Read the model definition and answer for the solid it produces. Units are mm, in the model's axes. A direction names the side the tool comes from. Coordinates: 2 decimals unless noted, no trailing zeros. Order: outer loops, then holes, each group sorted by start corner. A loop starts at its lowest first (then second) coordinate and runs counter-clockwise, first axis right, second up. Notation, with made-up numbers: M 86.5,72.25 L 131.5,72.25 A24 ccw 131.5,107.25 Z; hole C 29,68.5 d4. An arc over 180 degrees is marked long. Write each question's results on one line, items separated by ' | '.
```python
from build123d import *

# Parameters (mm, degrees)
BOSS_EXTRUDE1_DEPTH           = 10
M4_CLEARANCE_HOLE1_AT_2_COUNT = 2
M4_CLEARANCE_HOLE1_AT_2_PITCH = 112
SKETCH6_R                     = 3
CUT_EXTRUDE1_DEPTH            = 8
CUT_EXTRUDE1_DEPTH_BACK       = 6
FILLET1_R                     = 1


with BuildPart() as part:
    # Sketch1 → Boss-Extrude1 (new body)
    with BuildSketch(Plane(origin=(0, 0, 0), x_dir=(0, 0, -1), z_dir=(1, 0, 0))):
        with BuildLine():
            ThreePointArc((25, 57.609374237), (12.766583292, 61.488652214), (0, 62.8))
            ThreePointArc((0, 62.8), (-12.766583292, 61.488652214), (-25, 57.609374237))
            Line((-25, 57.609374237), (-25, 51.929182547))
            ThreePointArc((-25, 51.929182547), (-25.220795702, 51.145833095), (-25.818181818, 50.593097233))
            ThreePointArc((-25.818181818, 50.593097233), (-43.035646203, 37.069841595), (-53.859344034, 18.039153533))
            ThreePointArc((-53.859344034, 18.039153533), (-54.405495004, 17.298046479), (-55.281685866, 17.01553963))
            Line((-55.281685866, 17.01553963), (-59.5, 17.01553963))
            ThreePointArc((-59.5, 17.01553963), (-60.560660172, 16.576199802), (-61, 15.51553963))
            Line((-61, 15.51553963), (-61, 2.01553963))
            Line((-61, 2.01553963), (-50.76, 2.01553963))
            ThreePointArc((-50.76, 2.01553963), (0, 50.8), (50.76, 2.01553963))
            Line((50.76, 2.01553963), (61, 2.01553963))
            Line((61, 2.01553963), (61, 15.51553963))
            ThreePointArc((61, 15.51553963), (60.560660172, 16.576199802), (59.5, 17.01553963))
            Line((59.5, 17.01553963), (55.281685866, 17.01553963))
            ThreePointArc((55.281685866, 17.01553963), (54.405495004, 17.298046479), (53.859344034, 18.039153533))
            ThreePointArc((53.859344034, 18.039153533), (43.035646203, 37.069841595), (25.818181818, 50.593097233))
            ThreePointArc((25.818181818, 50.593097233), (25.220795702, 51.145833095), (25, 51.929182547))
            Line((25, 51.929182547), (25, 57.609374237))
        make_face()
    extrude(amount=BOSS_EXTRUDE1_DEPTH)

    # Sketch4 → M4 Clearance Hole1 (revolve, cut)
    with BuildSketch(Plane(origin=(5, 17.01553963, -56), x_dir=(0, 0, 1), z_dir=(1, 0, 0))):
        Polygon((0, 0), (0, 16.351936393), (2.25, 15), (2.25, 0), align=None)
    m4_clearance_hole1 = revolve(axis=Axis((5, 23.36553963, -56), (0, -1, 0)), mode=Mode.SUBTRACT)

    # M4 Clearance Hole1 at 2: M4 Clearance Hole1 ×2
    with Locations(*[(0, 0, i * M4_CLEARANCE_HOLE1_AT_2_PITCH) for i in range(1, M4_CLEARANCE_HOLE1_AT_2_COUNT)]):
        add(m4_clearance_hole1, mode=Mode.SUBTRACT)

    # Sketch6 → Cut-Extrude1 (cut, two sides)
    with BuildSketch(Plane(origin=(0, 17.01553963, 0), x_dir=(1, 0, 0), z_dir=(0, 1, 0))) as cut_extrude1_sk:
        with Locations((5, 56)):
            Circle(SKETCH6_R)
        with Locations((5, -56)):
            Circle(SKETCH6_R)
    extrude(amount=CUT_EXTRUDE1_DEPTH, mode=Mode.SUBTRACT)
    extrude(cut_extrude1_sk.sketch, amount=-CUT_EXTRUDE1_DEPTH_BACK, mode=Mode.SUBTRACT)

    # Fillet1
    fillet1_edges = [part.edges().sort_by_distance(p)[0] for p in [
        (5, 57.609374237, -25),
        (5, 57.609374237, 25),
    ]]
    fillet(fillet1_edges, radius=FILLET1_R)


solid = part.part
```
(1) The part is cut by section C-C, the plane y = 23.5. Write down the section's boundary in (x, z), then the cut area to 3 significant figures.
Conclusion:
outline: M 0,-51.71 L 10,-51.71 L 10,-45.04 L 0,-45.04 Z; M 0,45.04 L 10,45.04 L 10,51.71 L 0,51.71 Z | area: 133 mm²
(2) Given pin 1 (3 mm diameter, centred on x = 4, z = 57, fed in from +Y); pin 2 (8 mm diameter, centred on y = 32.5, z = 44, fed in from -X); pin 3 (1 mm diameter, centred on x = 2, z = -20.5, fed in from +Y); pin 4 (5.5 mm diameter, centred on x = 2.5, y = 53.5, fed in from -Z), each flat-ended and moving along its own axis, determine where each tip first touches the part or whether it passes through.
Conclusion:
pin 1: y = 11.02 | pin 2: x = 0 | pin 3: y = 59.53 | pin 4: z = -25.57
(3) The mould has two halves that part along X. Classify faces 4 (the cylindrical face through (4.901, 6.579, -58.248)), 5 (the flat face through (0, 51, 9)), 6 (the flat face through (2.7, 2.016, 54.8)), 7 (the flat face through (10, 51, 9)): pulls with the +X half, pulls with the -X half, needs draft (parallel to the pull), parting line crosses it, or undercut.
Conclusion:
face 4: undercut | face 5: pulls with the -X half | face 6: needs draft | face 7: pulls with the +X half
(4) The part is cut by section B-B, the plane y = 40. Write down the section's boundary in (x, z).
Conclusion:
outline: M 0,-40.33 L 10,-40.33 L 10,-31.32 L 0,-31.32 Z; M 0,31.32 L 10,31.32 L 10,40.33 L 0,40.33 Z
(5) For faces 1 (the cylindrical face through (4.901, 6.579, 53.752)), 2 (the flat face through (5, 54, -25)), 3 (the flat face through (5, 54, 25)), determine the directions among +Z, -Z, +X, -X, +Y, -Y from which every point of the face is accessible in a straight line to the end or side of a thin tool.
Conclusion:
face 1: +Y, -Y | face 2: -Z, +X, -X, +Y | face 3: +Z, +X, -X, +Y
(6) Straight lines are drawn through the part: line 1 (X direction, y = 15.35, z = -56); line 2 (X direction, y = 8.5, z = 56); line 3 (Z direction, x = 3.25, y = 12). For each, find the intervals that lie inside material, in ascending order.
Conclusion:
line 1: 0 to 2, 8 to 10 | line 2: 0 to 2.75, 7.25 to 10 | line 3: -61 to -58.44, -53.56 to -49.36, 49.36 to 53.56, 58.44 to 61
(7) The part is cut by section A-A, the plane x = 5. Count the separate pieces of the cut face and the enclosed holes in it, then the cut area to 3 significant figures.
Conclusion:
separate pieces: 3 | enclosed holes: 0 | area: 1,300 mm²
(8) The part is cut by section D-D, the plane z = -42.5. Write down the section's boundary in (x, y), then the cut area to 3 significant figures.
Conclusion:
outline: M 0,27.83 L 10,27.83 L 10,37.68 L 0,37.68 Z | area: 98.5 mm²
